```python
from build123d import *

# Parameters (mm, degrees)
SKETCH5_W         = 10
SKETCH5_H         = 17
EXTRUDE2_DEPTH    = 72.414284285
CIRPATTERN1_COUNT = 4


with BuildPart() as part:
    # Sketch1 → Revolve1 (revolve)
    with BuildSketch(Plane(origin=(0, 0, 0), x_dir=(0, 0, -1), z_dir=(1, 0, 0)), mode=Mode.PRIVATE) as revolve1_sk:
        with BuildLine():
            Line((0, 0), (-15, 0))
            Line((-15, 0), (-15, 19))
            Line((-15, 19), (-14, 20))
            Line((-14, 20), (-6, 20))
            ThreePointArc((-6, 20), (-5.292893219, 20.292893219), (-5, 21))
            Line((-5, 21), (-5, 50))
            Line((-5, 50), (0, 50))
            Line((0, 50), (0, 0))
        make_face()
    revolve(revolve1_sk.sketch.rotate(Axis((0, 0, 50), (0, 0, -1)), 90), axis=Axis((0, 0, 50), (0, 0, -1)))

    # Sketch5 → Extrude2 (cut, through all)
    with BuildSketch(Plane.XY.offset(5)):
        with Locations((45, 0)):
            Rectangle(SKETCH5_W, SKETCH5_H)
    extrude(amount=-EXTRUDE2_DEPTH, mode=Mode.SUBTRACT)

    # Sketch6 → Ø7.0 (7) Diameter Hole1 (revolve, cut)
    with BuildSketch(Plane(origin=(-30, 30, 5), x_dir=(0, -1, 0), z_dir=(1, 0, 0))):
        Polygon((0, 0), (0, 12.103012167), (3.5, 10), (3.5, 0), align=None)
    f_7_0_7_diameter_hole1 = revolve(axis=Axis((-30, 30, 11.35), (0, 0, -1)), mode=Mode.SUBTRACT)

    # CirPattern1: Ø7.0 (7) Diameter Hole1 ×4 about axis
    cirpattern1_axis = Axis((0, 0, 0), (0, 0, 1))
    for i in range(1, CIRPATTERN1_COUNT):
        add(f_7_0_7_diameter_hole1.rotate(cirpattern1_axis, i * 360 / CIRPATTERN1_COUNT), mode=Mode.SUBTRACT)


solid = part.part
```
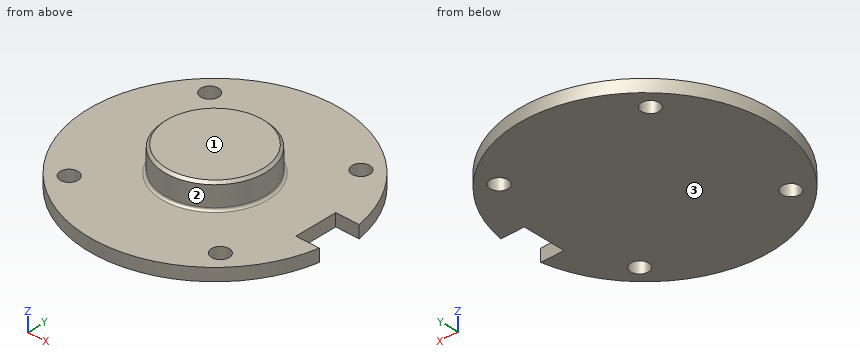
Model file for the job. Use its own axes, mm. Face numbers are marked on the shaded views. Give positions to 0.01 mm unless a question says otherwise; leave off trailing zeros. Loops run counter-clockwise (first coordinate to the right, second up) from the corner with the lowest first, then second, coordinate; pieces in that order, holes last. Notation, with made-up numbers: (57.25, -5) - (77.25, -5) arc R20 cw to (77.25, 28) - close; hole circle Ø7 at (-16.75, 33.25). An arc over 180 degrees is marked (long way). One line per item, written item: value. Start each with the question number.
1. Pull direction Z, two halves, no side cores. Call the marked faces 1, 2 and 3: pulls with the +Z half, pulls with the -Z half, needs draft (parallel to the pull), parting line crosses it, or undercut.
2. Pin check, flat tips, straight feed: pin 1 (5.5 mm diameter, centred on x = -30, y = 30, fed in from +Z); pin 2 (1.5 mm diameter, centred on x = 47, z = 1.5, fed in from +Y); pin 3 (1.5 mm diameter, centred on y = -10, z = 12, fed in from -X); pin 4 (5.5 mm diameter, centred on y = -1, z = 3.5, fed in from +X). Stop position of each tip, or through.
3. Slice it at D-D (y = 0). List the corners of the cut face in (x, z).
4. Slice it at A-A (x = -30). List the corners of the cut face in (y, z), plus the area to 3 significant figures.
5. Probe L1, parallel to X at y = 30, z = 2.75; L2, parallel to X at y = -32.5, z = 1.75. List the from-to ranges inside material, lowest first. Write a range as from..to.
6. Slice it at C-C (z = 3.25). List the corners of the cut face in (x, y), plus the area to 3 significant figures.
Solution:
1. face 1: pulls with the +Z half
1. face 2: needs draft
1. face 3: pulls with the -Z half
2. pin 1: passes through
2. pin 2: stops at y = 19
2. pin 3: stops at x = -17.73
2. pin 4: stops at x = 40
3. outline: (-50, 0) - (40, 0) - (40, 5) - (21, 5) arc R1 cw to (20, 6) - (20, 14) - (19, 15) - (-19, 15) - (-20, 14) - (-20, 6) arc R1 cw to (-21, 5) - (-50, 5) - close
4. outline: (-40, 0) - (-33.5, 0) - (-33.5, 5) - (-40, 5) - close; (-26.5, 0) - (26.5, 0) - (26.5, 5) - (-26.5, 5) - close; (33.5, 0) - (40, 0) - (40, 5) - (33.5, 5) - close
4. area: 330 mm^2
5. L1: x = -40..-33.5, -26.5..26.5, 33.5..40
5. L2: x = -38..-32.45, -27.55..27.55, 32.45..38
6. outline: (40, -8.5) - (40, 8.5) - (49.27, 8.5) arc R50 ccw (long way) to (49.27, -8.5) - close; hole circle Ø7 at (-30, -30); hole circle Ø7 at (-30, 30); hole circle Ø7 at (30, -30); hole circle Ø7 at (30, 30)
6. area: 7,530 mm^2
